```python
from build123d import *

# Parameters (mm, degrees)
SKETCH1_W           = 177.8
SKETCH1_H           = 38.1
BOSS_EXTRUDE1_DEPTH = 5.08
SKETCH2_W           = 11.43
SKETCH2_H           = 5.08
CUT_EXTRUDE1_DEPTH  = 5.08
SKETCH3_W           = 11.43
SKETCH3_H           = 5.08
CUT_EXTRUDE2_DEPTH  = 5.08
SKETCH4_W           = 17.78
SKETCH4_H           = 5.08
CUT_EXTRUDE3_DEPTH  = 5.08
LPATTERN1_COUNT     = 3
LPATTERN1_PITCH     = 43.18
SKETCH5_W           = 40.5765
SKETCH5_H           = 19.812
CUT_EXTRUDE4_DEPTH  = 5.08
SKETCH6_W           = 5.08
SKETCH6_H           = 12.7
CUT_EXTRUDE5_DEPTH  = 5.08
SKETCH7_W           = 11.43
SKETCH7_H           = 5.08
SKETCH7_W_2         = 17.78
CUT_EXTRUDE6_DEPTH  = 5.08
SKETCH8_W           = 17.78
SKETCH8_H           = 5.08
CUT_EXTRUDE7_DEPTH  = 5.08
LPATTERN2_COUNT     = 2
LPATTERN2_PITCH     = 43.18
SKETCH9_W           = 5.08
SKETCH9_H           = 12.7
CUT_EXTRUDE8_DEPTH  = 5.08
SKETCH10_R          = 2.159
CUT_EXTRUDE9_DEPTH  = 5.08


with BuildPart() as part:
    # Sketch1 → Boss-Extrude1 (new body)
    with BuildSketch(Plane(origin=(0, 0, 0), x_dir=(1, 0, 0), z_dir=(0, 1, 0))):
        with Locations((-88.9, -19.05)):
            Rectangle(SKETCH1_W, SKETCH1_H)
    extrude(amount=BOSS_EXTRUDE1_DEPTH)

    # Sketch2 → Cut-Extrude1 (cut)
    with BuildSketch(Plane(origin=(0, 5.08, 0), x_dir=(1, 0, 0), z_dir=(0, 1, 0))):
        with Locations((-172.085, -35.56)):
            Rectangle(SKETCH2_W, SKETCH2_H)
    extrude(amount=-CUT_EXTRUDE1_DEPTH, mode=Mode.SUBTRACT)

    # Sketch3 → Cut-Extrude2 (cut)
    with BuildSketch(Plane(origin=(0, 5.08, 0), x_dir=(1, 0, 0), z_dir=(0, 1, 0))):
        with Locations((-5.715, -35.56)):
            Rectangle(SKETCH3_W, SKETCH3_H)
    extrude(amount=-CUT_EXTRUDE2_DEPTH, mode=Mode.SUBTRACT)

    # Sketch4 → Cut-Extrude3 (cut)
    with BuildSketch(Plane(origin=(0, 5.08, 0), x_dir=(1, 0, 0), z_dir=(0, 1, 0))):
        with Locations((-132.08, -35.56)):
            Rectangle(SKETCH4_W, SKETCH4_H)
    cut_extrude3 = extrude(amount=-CUT_EXTRUDE3_DEPTH, mode=Mode.SUBTRACT)

    # LPattern1: Cut-Extrude3 ×3
    with Locations(*[(i * LPATTERN1_PITCH, 0, 0) for i in range(1, LPATTERN1_COUNT)]):
        add(cut_extrude3, mode=Mode.SUBTRACT)

    # Sketch5 → Cut-Extrude4 (cut)
    with BuildSketch(Plane(origin=(0, 5.08, 0), x_dir=(1, 0, 0), z_dir=(0, 1, 0))):
        with Locations((-55.84825, -23.114)):
            Rectangle(SKETCH5_W, SKETCH5_H)
    extrude(amount=-CUT_EXTRUDE4_DEPTH, mode=Mode.SUBTRACT)

    # Sketch6 → Cut-Extrude5 (cut)
    with BuildSketch(Plane(origin=(0, 0, 0), x_dir=(-1, 0, 0), z_dir=(0, -1, 0))):
        with Locations((2.54, -16.51)):
            Rectangle(SKETCH6_W, SKETCH6_H)
    extrude(amount=-CUT_EXTRUDE5_DEPTH, mode=Mode.SUBTRACT)

    # Sketch7 → Cut-Extrude6 (cut)
    with BuildSketch(Plane(origin=(0, 5.08, 0), x_dir=(1, 0, 0), z_dir=(0, 1, 0))):
        with Locations((-172.085, -2.54)):
            Rectangle(SKETCH7_W, SKETCH7_H)
        with Locations((-132.08, -2.54)):
            Rectangle(SKETCH7_W_2, SKETCH7_H)
        with Locations((-5.715, -2.54)):
            Rectangle(SKETCH7_W, SKETCH7_H)
    extrude(amount=-CUT_EXTRUDE6_DEPTH, mode=Mode.SUBTRACT)

    # Sketch8 → Cut-Extrude7 (cut)
    with BuildSketch(Plane(origin=(0, 5.08, 0), x_dir=(1, 0, 0), z_dir=(0, 1, 0))):
        with Locations((-88.9, -2.54)):
            Rectangle(SKETCH8_W, SKETCH8_H)
    cut_extrude7 = extrude(amount=-CUT_EXTRUDE7_DEPTH, mode=Mode.SUBTRACT)

    # LPattern2: Cut-Extrude7 ×2
    with Locations(*[(i * LPATTERN2_PITCH, 0, 0) for i in range(1, LPATTERN2_COUNT)]):
        add(cut_extrude7, mode=Mode.SUBTRACT)

    # Sketch9 → Cut-Extrude8 (cut)
    with BuildSketch(Plane(origin=(0, 5.08, 0), x_dir=(1, 0, 0), z_dir=(0, 1, 0))):
        with Locations((-175.26, -16.51)):
            Rectangle(SKETCH9_W, SKETCH9_H)
    extrude(amount=-CUT_EXTRUDE8_DEPTH, mode=Mode.SUBTRACT)

    # Sketch10 → Cut-Extrude9 (cut)
    with BuildSketch(Plane.XZ):
        with Locations((-80.9625, 18.542)):
            Circle(SKETCH10_R)
        with Locations((-80.9625, 28.448)):
            Circle(SKETCH10_R)
        with Locations((-30.226, 28.448)):
            Circle(SKETCH10_R)
        with Locations((-30.226, 18.542)):
            Circle(SKETCH10_R)
    extrude(amount=-CUT_EXTRUDE9_DEPTH, mode=Mode.SUBTRACT)


solid = part.part
```
Can you work these out from the model? Positions are in its coordinate system, mm. A direction names the side the tool comes from. Round coordinates to 2 decimals unless told otherwise and drop trailing zeros. Order: outer loops, then holes, each group sorted by start corner. A loop starts at its lowest first (then second) coordinate and runs counter-clockwise, first axis right, second up. Notation, with made-up numbers: (-16, 43.25) -> (-12, 43.25) arc R27 cw to (-12, 78.25) -> close; hole circle Ø6 at (88, 75). An arc over 180 degrees is marked (long way). Return JSON: item names as keys, results as strings. Group by question number.
1. If we section it at A-A, the plane z = 36: Write out the boundary of the cut face in (x, y).
2. We'd pull the mould along Z, two halves only. Please class faces 1 (the face through (-54.61, 3, 3)), 2 (the face through (-175, 3, 22.86)), 3 (the face through (-132, 3, 5.08)), 4 (the face through (-67, 3, 38.1)): released by +Z, released by -Z, zero draft, split by the parting line, or undercut.
3. If we section it at B-B, the plane x = -94: Write out the boundary of the cut face in (y, z), then the cut area to 3 significant figures.
4. I need wall thicknesses on line 1 (X direction, y = 1.05, z = 18.5); line 2 (X direction, y = 2.2, z = 3); line 3 (X direction, y = 2.05, z = 21). Which ranges of each line are inside material? Lowest first, please. Write a range as [from, to].
5. Will these pins go through, and if not, where does the flat tip stop? pin 1 (4 mm diameter, centred on x = -29, z = 28.5, fed in from -Y); pin 2 (1.5 mm diameter, centred on y = 1.5, z = 1.5, fed in from -X); pin 3 (1.5 mm diameter, centred on x = -49.5, y = 3.5, fed in from +Z); pin 4 (1.5 mm diameter, centred on y = 2, z = 36, fed in from +X).
6. If we section it at C-C, the plane y = 2.5: Count the separate pieces of the cut face and the enclosed holes in it, then the cut area to 3 significant figures.
7. Which directions (+Z, -Z, +X, -X, +Y, -Y) give clear straight access to the entire face, cutting with the end or side of a thin tool? Please do faces 5 (the face through (-123.19, 3, 3)), 6 (the face through (-175, 3, 10.16)), 7 (the face through (-166.37, 3, 3)), 8 (the face through (-132, 3, 33.02)), 9 (the face through (-6, 3, 5.08)).
Output values:
{
 "1": {"outline": "(-166.37, 0) -> (-140.97, 0) -> (-140.97, 5.08) -> (-166.37, 5.08) -> close; (-123.19, 0) -> (-97.79, 0) -> (-97.79, 5.08) -> (-123.19, 5.08) -> close; (-80.01, 0) -> (-54.61, 0) -> (-54.61, 5.08) -> (-80.01, 5.08) -> close; (-36.83, 0) -> (-11.43, 0) -> (-11.43, 5.08) -> (-36.83, 5.08) -> close"},
 "2": {"face 1": "zero draft", "face 2": "undercut", "face 3": "released by -Z", "face 4": "released by +Z"},
 "3": {"outline": "(0, 5.08) -> (5.08, 5.08) -> (5.08, 33.02) -> (0, 33.02) -> close", "area": "142 mm²"},
 "4": {"line 1": "[-172.72, -83.12], [-78.8, -76.14], [-35.56, -32.38], [-28.07, -5.08]", "line 2": "[-166.37, -140.97], [-123.19, -97.79], [-80.01, -54.61], [-36.83, -11.43]", "line 3": "[-172.72, -76.14], [-35.56, -5.08]"},
 "5": {"pin 1": "y = 0", "pin 2": "x = -166.37", "pin 3": "z = 13.21", "pin 4": "x = -11.43"},
 "6": {"separate pieces": "1", "enclosed holes": "4", "area": "5,010 mm²"},
 "7": {"face 5": "-Z, +Y, -Y", "face 6": "-X, +Y, -Y", "face 7": "-Z, -X, +Y, -Y", "face 8": "+Z, +Y, -Y", "face 9": "-Z, +X, +Y, -Y"}
}
